```python
from build123d import *

# Parameters (mm, degrees)
BOSS_EXTRUDE1_DEPTH     = 19.05
SKETCH3_W               = 50.8
SKETCH3_H               = 25.4
CUT_EXTRUDE2_DEPTH      = 985.608197724
SKETCH4_W               = 609.6
SKETCH4_H               = 12.7
CUT_EXTRUDE3_DEPTH      = 985.608197724
CUT_EXTRUDE4_DEPTH      = 985.608197724
CUT_EXTRUDE4_DEPTH_BACK = 985.608197724
SKETCH5_W               = 533.4
SKETCH5_H               = 224.282
CUT_EXTRUDE5_DEPTH      = 985.608197724
CUT_EXTRUDE5_DEPTH_BACK = 985.608197724
SKETCH6_W               = 1348.924846149
SKETCH6_H               = 423.84329992
FILLET1_R               = 3.175


with BuildPart() as part:
    # Sketch1 → Boss-Extrude1 (new body)
    with BuildSketch(Plane.XY):
        with BuildLine():
            Line((0, 0), (0, 85.725))
            ThreePointArc((0, 85.725), (3.175, 88.9), (0, 92.075))
            Line((0, 92.075), (-19.05, 92.075))
            Line((-19.05, 92.075), (-19.05, 111.125))
            Line((-19.05, 111.125), (0, 111.125))
            ThreePointArc((0, 111.125), (3.175, 114.3), (0, 117.475))
            Line((0, 117.475), (0, 206.375))
            ThreePointArc((0, 206.375), (3.175, 209.55), (0, 212.725))
            Line((0, 212.725), (-19.05, 212.725))
            Line((-19.05, 212.725), (-19.05, 231.775))
            Line((-19.05, 231.775), (0, 231.775))
            ThreePointArc((0, 231.775), (3.175, 234.95), (0, 238.125))
            Line((0, 238.125), (0, 327.025))
            ThreePointArc((0, 327.025), (3.175, 330.2), (0, 333.375))
            Line((0, 333.375), (-19.05, 333.375))
            Line((-19.05, 333.375), (-19.05, 352.425))
            Line((-19.05, 352.425), (0, 352.425))
            ThreePointArc((0, 352.425), (3.175, 355.6), (0, 358.775))
            Line((0, 358.775), (0, 447.675))
            ThreePointArc((0, 447.675), (3.175, 450.85), (0, 454.025))
            Line((0, 454.025), (-19.05, 454.025))
            Line((-19.05, 454.025), (-19.05, 473.075))
            Line((-19.05, 473.075), (0, 473.075))
            ThreePointArc((0, 473.075), (3.175, 476.25), (0, 479.425))
            Line((0, 479.425), (0, 568.325))
            ThreePointArc((0, 568.325), (3.175, 571.5), (0, 574.675))
            Line((0, 574.675), (-19.05, 574.675))
            Line((-19.05, 574.675), (-19.05, 593.725))
            Line((-19.05, 593.725), (0, 593.725))
            ThreePointArc((0, 593.725), (3.175, 596.9), (0, 600.075))
            Line((0, 600.075), (0, 688.975))
            ThreePointArc((0, 688.975), (3.175, 692.15), (0, 695.325))
            Line((0, 695.325), (-19.05, 695.325))
            Line((-19.05, 695.325), (-19.05, 714.375))
            Line((-19.05, 714.375), (0, 714.375))
            ThreePointArc((0, 714.375), (3.175, 717.55), (0, 720.725))
            Line((0, 720.725), (0, 757.555))
            Line((0, 757.555), (609.6, 757.555))
            Line((609.6, 757.555), (609.6, 720.725))
            ThreePointArc((609.6, 720.725), (606.425, 717.55), (609.6, 714.375))
            Line((609.6, 714.375), (628.65, 714.375))
            Line((628.65, 714.375), (628.65, 695.325))
            Line((628.65, 695.325), (609.6, 695.325))
            ThreePointArc((609.6, 695.325), (606.425, 692.15), (609.6, 688.975))
            Line((609.6, 688.975), (609.6, 600.075))
            ThreePointArc((609.6, 600.075), (606.425, 596.9), (609.6, 593.725))
            Line((609.6, 593.725), (628.65, 593.725))
            Line((628.65, 593.725), (628.65, 574.675))
            Line((628.65, 574.675), (609.6, 574.675))
            ThreePointArc((609.6, 574.675), (606.425, 571.5), (609.6, 568.325))
            Line((609.6, 568.325), (609.6, 479.425))
            ThreePointArc((609.6, 479.425), (606.425, 476.25), (609.6, 473.075))
            Line((609.6, 473.075), (628.65, 473.075))
            Line((628.65, 473.075), (628.65, 454.025))
            Line((628.65, 454.025), (609.6, 454.025))
            ThreePointArc((609.6, 454.025), (606.425, 450.85), (609.6, 447.675))
            Line((609.6, 447.675), (609.6, 358.775))
            ThreePointArc((609.6, 358.775), (606.425, 355.6), (609.6, 352.425))
            Line((609.6, 352.425), (628.65, 352.425))
            Line((628.65, 352.425), (628.65, 333.375))
            Line((628.65, 333.375), (609.6, 333.375))
            ThreePointArc((609.6, 333.375), (606.425, 330.2), (609.6, 327.025))
            Line((609.6, 327.025), (609.6, 238.125))
            ThreePointArc((609.6, 238.125), (606.425, 234.95), (609.6, 231.775))
            Line((609.6, 231.775), (628.65, 231.775))
            Line((628.65, 231.775), (628.65, 212.725))
            Line((628.65, 212.725), (609.6, 212.725))
            ThreePointArc((609.6, 212.725), (606.425, 209.55), (609.6, 206.375))
            Line((609.6, 206.375), (609.6, 117.475))
            ThreePointArc((609.6, 117.475), (606.425, 114.3), (609.6, 111.125))
            Line((609.6, 111.125), (628.65, 111.125))
            Line((628.65, 111.125), (628.65, 92.075))
            Line((628.65, 92.075), (609.6, 92.075))
            ThreePointArc((609.6, 92.075), (606.425, 88.9), (609.6, 85.725))
            Line((609.6, 85.725), (609.6, 0))
            Line((609.6, 0), (0, 0))
        make_face()
    extrude(amount=BOSS_EXTRUDE1_DEPTH)

    # Sketch3 → Cut-Extrude2 (cut, through all)
    with BuildSketch(Plane.XY.offset(19.05)):
        with Locations((104.775, 501.65)):
            Rectangle(SKETCH3_W, SKETCH3_H)
        with Locations((104.775, 381)):
            Rectangle(SKETCH3_W, SKETCH3_H)
        with Locations((104.775, 260.35)):
            Rectangle(SKETCH3_W, SKETCH3_H)
        with Locations((104.775, 139.7)):
            Rectangle(SKETCH3_W, SKETCH3_H)
        with Locations((304.8, 139.7)):
            Rectangle(SKETCH3_W, SKETCH3_H)
        with Locations((304.8, 260.35)):
            Rectangle(SKETCH3_W, SKETCH3_H)
        with Locations((304.8, 381)):
            Rectangle(SKETCH3_W, SKETCH3_H)
        with Locations((304.8, 501.65)):
            Rectangle(SKETCH3_W, SKETCH3_H)
        with Locations((504.825, 501.65)):
            Rectangle(SKETCH3_W, SKETCH3_H)
        with Locations((504.825, 381)):
            Rectangle(SKETCH3_W, SKETCH3_H)
        with Locations((504.825, 260.35)):
            Rectangle(SKETCH3_W, SKETCH3_H)
        with Locations((504.825, 139.7)):
            Rectangle(SKETCH3_W, SKETCH3_H)
    extrude(amount=-CUT_EXTRUDE2_DEPTH, mode=Mode.SUBTRACT)

    # Sketch4 → Cut-Extrude3 (cut, through all)
    with BuildSketch(Plane.XY.offset(19.05)):
        with Locations((304.8, 6.35)):
            Rectangle(SKETCH4_W, SKETCH4_H)
    extrude(amount=-CUT_EXTRUDE3_DEPTH, mode=Mode.SUBTRACT)

    # Sketch5 → Cut-Extrude4 (cut, two sides: drawn at the far end of the back side and taken through both)
    with BuildSketch(Plane.XY.offset(19.05).offset(-CUT_EXTRUDE4_DEPTH_BACK)):
        with Locations((304.8, 645.414)):
            Rectangle(SKETCH5_W, SKETCH5_H)
    extrude(amount=CUT_EXTRUDE4_DEPTH + CUT_EXTRUDE4_DEPTH_BACK, mode=Mode.SUBTRACT)

    # Sketch6 → Cut-Extrude5 (cut, two sides: drawn at the far end of the back side and taken through both)
    with BuildSketch(Plane.XY.offset(19.05).offset(-CUT_EXTRUDE5_DEPTH_BACK)):
        with Locations((467.467327316, 745.19464996)):
            Rectangle(SKETCH6_W, SKETCH6_H)
    extrude(amount=CUT_EXTRUDE5_DEPTH + CUT_EXTRUDE5_DEPTH_BACK, mode=Mode.SUBTRACT)

    # Fillet1
    fillet1_edges = [part.edges().sort_by_distance(p)[0] for p in [
        (530.225, 488.95, 9.525),
        (479.425, 488.95, 9.525),
        (479.425, 514.35, 9.525),
        (530.225, 514.35, 9.525),
        (330.2, 514.35, 9.525),
        (330.2, 488.95, 9.525),
        (279.4, 488.95, 9.525),
        (279.4, 514.35, 9.525),
        (330.2, 393.7, 9.525),
        (330.2, 368.3, 9.525),
        (279.4, 368.3, 9.525),
        (279.4, 393.7, 9.525),
        (330.2, 273.05, 9.525),
        (330.2, 247.65, 9.525),
        (279.4, 247.65, 9.525),
        (279.4, 273.05, 9.525),
        (330.2, 152.4, 9.525),
        (330.2, 127, 9.525),
        (279.4, 127, 9.525),
        (279.4, 152.4, 9.525),
        (130.175, 127, 9.525),
        (79.375, 127, 9.525),
        (79.375, 152.4, 9.525),
        (130.175, 152.4, 9.525),
        (130.175, 247.65, 9.525),
        (79.375, 247.65, 9.525),
        (79.375, 273.05, 9.525),
        (130.175, 273.05, 9.525),
        (130.175, 368.3, 9.525),
        (79.375, 368.3, 9.525),
        (79.375, 393.7, 9.525),
        (130.175, 393.7, 9.525),
        (530.225, 368.3, 9.525),
        (479.425, 368.3, 9.525),
        (479.425, 393.7, 9.525),
        (530.225, 393.7, 9.525),
        (530.225, 247.65, 9.525),
        (479.425, 247.65, 9.525),
        (479.425, 273.05, 9.525),
        (530.225, 273.05, 9.525),
        (530.225, 127, 9.525),
        (479.425, 127, 9.525),
        (479.425, 152.4, 9.525),
        (530.225, 152.4, 9.525),
        (130.175, 488.95, 9.525),
        (79.375, 488.95, 9.525),
        (79.375, 514.35, 9.525),
        (130.175, 514.35, 9.525),
    ]]
    fillet(fillet1_edges, radius=FILLET1_R)


solid = part.part
```
The listing builds one solid part. Answer for the finished solid, in the listing's coordinates (mm). A direction names the side the tool comes from. Give positions to 0.01 mm unless a question says otherwise; leave off trailing zeros. One line per item, written item: value.
Q1. Flat-ended cylindrical pins translate along their axes: P1, Ø5.5, axis at y = 137.5, z = 5.5, coming from the -X side; P2, Ø1, axis at y = 129, z = 8.5, coming from the +X side. Find the tip coordinate at first contact, or state that the pin passes through.
Working result:
P1: stops at x = 0
P2: stops at x = 609.6
Q2. For faces 1 (the face through (609.6, 507, 9)), 2 (the face through (130.175, 381, 10)), 3 (the face through (619, 212.725, 9)), 4 (the face through (301, 12.7, 10)), determine the directions among +Z, -Z, +X, -X, +Y, -Y from which every point of the face is accessible in a straight line to the end or side of a thin tool.
Working result:
face 1: +Z, -Z, +X, +Y
face 2: +Z, -Z
face 3: +Z, -Z, +X
face 4: +Z, -Z, +X, -X, -Y
Q3. Determine the mould class of faces 5 (the face through (609.6, 50, 9)), 6 (the face through (-10, 473.075, 9)), 7 (the face through (479.425, 502, 10)) for opening direction Y: +Y half, -Y half, draft (parallel to the pull), parting line (faces both ways), or undercut.
Working result:
face 5: draft
face 6: +Y half
face 7: undercut
Q4. Find the intervals of material crossed by line 1 (Y direction, x = 327.5, z = 13.5); line 2 (X direction, y = 145.5, z = 9.25) (3 decimals); line 3 (Y direction, x = 125, z = 3.75), in increasing order. Write a range as from..to.
Working result:
line 1: y = 12.7..127.04, 152.36..247.69, 273.01..368.34, 393.66..488.99, 514.31..533.27
line 2: x = 0..79.375, 130.175..279.4, 330.2..479.425, 530.225..609.6
line 3: y = 12.7..127, 152.4..247.65, 273.05..368.3, 393.7..488.95, 514.35..533.27
Q5. A cutting plane is placed at A-A on z = 9.5. Give the number of separate pieces and of enclosed holes in the cut face, then the cut area to 3 significant figures.
Working result:
separate pieces: 1
enclosed holes: 12
area: 305,000 mm^2
